Autodesk Inventor part; units mm, degrees
ref_plane "YZ Plane" through (0, 0, 0) normal (1, 0, 0) x (0, 1, 0)
ref_plane "XZ Plane" through (0, 0, 0) normal (0, 1, 0) x (-1, 0, 0)
ref_plane "XY Plane" through (0, 0, 0) normal (0, 0, 1) x (1, 0, 0)
sketch "Sketch1" plane through (0, 0, 0) normal (1, 0, 0) x (0, 1, 0)
  line L0 (0, 0) -> (152.4, 0)
  line L1 (152.4, 0) -> (152.4, 19.05)
  line L2 (152.4, 19.05) -> (0, 19.05)
  line L3 (0, 19.05) -> (0, 0)
  circle A0 centre (12.7, 9.525) radius 3.175
  circle A1 centre (22.225, 9.525) radius 3.175
  circle A2 centre (31.75, 9.525) radius 3.175
  circle A3 centre (41.275, 9.525) radius 3.175
  circle A4 centre (50.8, 9.525) radius 3.175
  circle A5 centre (60.325, 9.525) radius 3.175
  circle A6 centre (69.85, 9.525) radius 3.175
  circle A7 centre (79.375, 9.525) radius 3.175
  circle A8 centre (88.9, 9.525) radius 3.175
  circle A9 centre (98.425, 9.525) radius 3.175
  circle A10 centre (107.95, 9.525) radius 3.175
  circle A11 centre (117.475, 9.525) radius 3.175
  circle A12 centre (127, 9.525) radius 3.175
  circle A13 centre (136.525, 9.525) radius 3.175
  dimension "d0" = 19.05
  dimension "d1" = 152.4
  dimension "d2" = 6.35
  dimension "d3" = 12.7
  dimension "d4" = 9.525
  dimension "d7" = 9.525
extrude "Extrusion1" add sketch "Sketch1" along normal blind 6.35
properties part number "Handle-Cart Link"
Verification items for the finished model (mm, model axes). Round coordinates to 2 decimals unless told otherwise and drop trailing zeros. Write each loop counter-clockwise with the first axis right and the second up, starting at its lowest first coordinate (ties: lowest second). Pieces come first, ordered by that corner, then holes.
(1) Mould release check, pull along Y, two halves, no side actions. Record for faces 1 (the flat face through (6.35, 75, 10)), 2 (the flat face through (3, 152.4, 9)), 3 (the cylindrical face through (3.131, 114.303, 9.385)): pulls with the +Y half, pulls with the -Y half, needs draft (parallel to the pull), parting line crosses it, or undercut.
Returned:
face 1: needs draft
face 2: pulls with the +Y half
face 3: undercut
(2) Material ranges on line 1 (Z direction, x = 3.5, y = 79); line 2 (Z direction, x = 3, y = 77.5), recorded low to high.
Returned:
line 1: z = 0 to 6.37, 12.68 to 19.05
line 2: z = 0 to 6.96, 12.09 to 19.05
(3) Section check A-A (x = 4.5). Give the number of separate pieces and of enclosed holes in the cut face, plus the area to 3 significant figures.
Returned:
separate pieces: 1
enclosed holes: 14
area: 2,460 mm2
(4) Section check B-B (y = 50.8). Enter the section's corners in (x, z), plus the area to 3 significant figures.
Returned:
outline: (0, 0) - (6.35, 0) - (6.35, 6.35) - (0, 6.35) - close; (0, 12.7) - (6.35, 12.7) - (6.35, 19.05) - (0, 19.05) - close
area: 80.6 mm2
(5) Depth check by flat-ended pin: pin 1 Ø3 at (y, z) = (101, 9) entering from +X. Enter the tip coordinate at first touch or a pass-through.
Returned:
pin 1: stops at x = 6.35
(6) Section check C-C (y = 127.5). Enter the section's corners in (x, z), plus the area to 3 significant figures.
Returned:
outline: (0, 0) - (6.35, 0) - (6.35, 6.39) - (0, 6.39) - close; (0, 12.66) - (6.35, 12.66) - (6.35, 19.05) - (0, 19.05) - close
area: 81.1 mm2
